Input: part model. Units: mm. Frame: model coordinates. Face numbers are marked on the shaded views. A direction names the side the tool comes from. Coordinates: 2 decimals unless noted, no trailing zeros. Loops run counter-clockwise (first coordinate to the right, second up) from the corner with the lowest first, then second, coordinate; pieces in that order, holes last. Notation, with made-up numbers: (82, 2.5) - (105, 2.5) arc R18 ccw to (105, 35.5) - close; hole circle Ø4 at (-13, 75). An arc over 180 degrees is marked (long way). Use a Markdown table: item, result. Add a question column.
1. Ray query, L1, parallel to Z at x = -23.75, y = 4.75; L2, parallel to X at y = 11.25, z = -36.5; L3, parallel to Y at x = -4, z = -20.5. Return the intervals inside material, ascending. Write a range as [from, to].
2. Contact query for flat-ended pins moving along their axis: P1, Ø3, axis at x = -13.5, z = -14, coming from the +Y side; P2, Ø3, axis at x = -16, y = 11, coming from the -Z side; P3, Ø0.9, axis at x = -20, y = 5, coming from the +Z side. Output: stop coordinate, or through.
3. Section query A-A on y = 5. Return the cut outline in (x, z), then the cut area to 3 significant figures.
4. Section query C-C on x = -17.75. Return the cut outline in (y, z), then the cut area to 3 significant figures.
5. Section query D-D on y = 11.5. Return the cut outline in (x, z), then the cut area to 3 significant figures.
6. Draft query along X for the marked faces 1, 2 and 3. Return one class per face: released by +X, released by -X, zero draft, split by the parting line, or undercut.
7. Access query for the marked faces 4, 5, 6, 7 and 8. Directions: +Z, -Z, +X, -X, +Y, -Y. A direction counts if a zero-diameter tool reaches every point of the face in a straight line with its end or side. Return the directions, or none.
8. Section query B-B on z = -27.5. Return the cut outline in (x, y).
Autodesk Inventor part; units mm, degrees
ref_plane "YZ Plane" through (0, 0, 0) normal (1, 0, 0) x (0, 1, 0)
ref_plane "XZ Plane" through (0, 0, 0) normal (0, 1, 0) x (-1, 0, 0)
ref_plane "XY Plane" through (0, 0, 0) normal (0, 0, 1) x (1, 0, 0)
sketch "Sketch1" plane through (0, 0, 0) normal (1, 0, 0) x (0, 1, 0)
  line L0 (0, 0) -> (30, 0)
  line L1 (30, 0) -> (30, -11)
  line L2 (30, -11) -> (21, -20)
  line L3 (21, -20) -> (19, -20)
  line L4 (19, -20) -> (19, -22)
  line L5 (19, -22) -> (21, -22)
  line L6 (21, -22) -> (30, -31)
  line L7 (30, -31) -> (30, -42)
  line L8 (30, -42) -> (0, -42)
  line L9 (0, 0) -> (0, -42)
  dimension "d5" = 42
  dimension "d6" = 30
  dimension "d7" = 2
  dimension "d8" = 11
  dimension "d9" = 2
  dimension "d10" = 2
  dimension "d17" = 20
  dimension "d18" = 11
extrude "Extrusion1" add sketch "Sketch1" against normal blind 30
sketch "Sketch2" plane through (0, 30, 0) normal (0, 1, 0) x (1, 0, 0)
  line L0 (0, 0) -> (-30, 0)
  line L1 (-25, 0) -> (-25, 6)
  line L2 (-25, 6) -> (-5, 6)
  line L3 (-5, 6) -> (-5, 0)
  line L4 (-30, 0) -> (-30, 11)
  line L5 (0, 11) -> (0, 0)
  line L6 (-25, 0) -> (-5, 0)
  line L7 (0, 42) -> (-30, 42)
  line L8 (-5, 42) -> (-5, 36)
  line L9 (-5, 36) -> (-25, 36)
  line L10 (-25, 36) -> (-25, 42)
  line L11 (-30, 31) -> (-30, 42)
  line L12 (0, 42) -> (0, 31)
  dimension "d13" = 5
  dimension "d14" = 5
  dimension "d21" = 30
  dimension "d22" = 6
  dimension "d23" = 5
  dimension "d24" = 5
extrude "Extrusion2" cut sketch "Sketch2" against normal blind 30 contours L0 L1 L2 L3
extrude "Extrusion3" cut sketch "Sketch2" against normal blind 30 contours L8 L9 L10 L7
sketch "Sketch4" plane through (0, 0, 0) normal (1, 0, 0) x (0, 0, -1)
  line L0 (42, 0) -> (0, 0)
  line L1 (15.5, 0) -> (15.5, 4)
  line L2 (15.5, 4) -> (13, 4)
  line L3 (13, 4) -> (13, 7)
  line L4 (13, 7) -> (29, 7)
  line L5 (29, 7) -> (29, 4)
  line L6 (29, 4) -> (26.5, 4)
  line L7 (26.5, 4) -> (26.5, 0)
  line L8 (0, 30) -> (0, 0)
  line L9 (42, 0) -> (42, 30)
  line L10 (15.5, 0) -> (26.5, 0)
  dimension "d27" = 15.5
  dimension "d28" = 15.5
  dimension "d29" = 2.5
  dimension "d30" = 2.5
  dimension "d31" = 3
  dimension "d32" = 4
extrude "Extrusion4" cut sketch "Sketch4" against normal blind 30
properties part number "peca2"
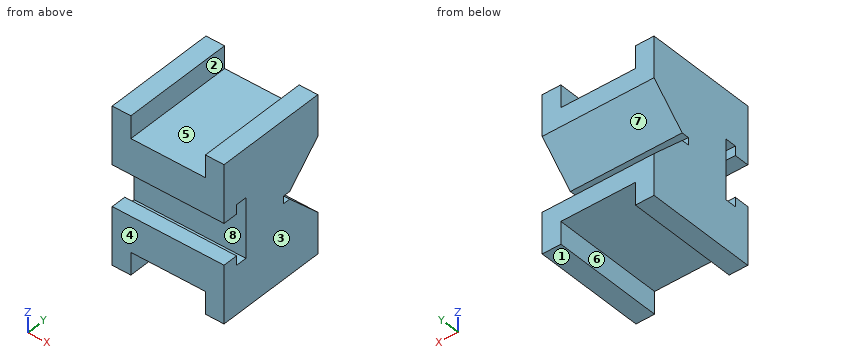
Resolved:
| question | item | result |
|---|---|---|
| 1 | L1 | [-36, -29], [-13, -6] |
| 1 | L2 | [-30, -25], [-5, 0] |
| 1 | L3 | [7, 19] |
| 2 | P1 | y = 28.5 |
| 2 | P2 | z = -36 |
| 2 | P3 | z = -6 |
| 3 | outline | (-30, -42) - (-25, -42) - (-25, -36) - (-5, -36) - (-5, -42) - (0, -42) - (0, -29) - (-30, -29) - close; (-30, -13) - (0, -13) - (0, 0) - (-5, 0) - (-5, -6) - (-25, -6) - (-25, 0) - (-30, 0) - close |
| 3 | area | 540 mm² |
| 4 | outline | (0, -36) - (30, -36) - (30, -31) - (21, -22) - (19, -22) - (19, -20) - (21, -20) - (30, -11) - (30, -6) - (0, -6) - (0, -15.5) - (4, -15.5) - (4, -13) - (7, -13) - (7, -29) - (4, -29) - (4, -26.5) - (0, -26.5) - close |
| 4 | area | 705 mm² |
| 5 | outline | (-30, -42) - (-25, -42) - (-25, -36) - (-5, -36) - (-5, -42) - (0, -42) - (0, 0) - (-5, 0) - (-5, -6) - (-25, -6) - (-25, 0) - (-30, 0) - close |
| 5 | area | 1,020 mm² |
| 6 | face 1 | zero draft |
| 6 | face 2 | undercut |
| 6 | face 3 | released by +X |
| 7 | face 4 | +Z, -Z, +X, -X, -Y |
| 7 | face 5 | +Z, +Y, -Y |
| 7 | face 6 | -Z, +Y, -Y |
| 7 | face 7 | +X, -X, +Y |
| 7 | face 8 | +X, -X |
| 8 | outline | (-30, 0) - (0, 0) - (0, 4) - (-30, 4) - close; (-30, 7) - (0, 7) - (0, 26.5) - (-30, 26.5) - close |
